For this review, use the dimensioned drawing (mm, ordinates from the lowest corner) and the shaded views. Round coordinates to 2 decimals unless told otherwise and drop trailing zeros. Loops run counter-clockwise (first coordinate to the right, second up) from the corner with the lowest first, then second, coordinate; pieces in that order, holes last. Notation, with made-up numbers: M 19,62 L 78,62 A16 cw 78,90 Z; hole C 2,-1.5 d10. An arc over 180 degrees is marked long. Answer as a JSON object with one key per item and string values. Group by question number.
Item 1: Consider section C-C (z = 2.7). Give the boundary of the cut face in (x, y).
Item 2: The part is to be moulded in two halves that separate along Y. For the marked faces 1 and 2, say which applies: +Y half, -Y half, draft (parallel to the pull), parting line (faces both ways), or undercut.
Item 3: Insertion check: P1, Ø1, axis at y = 35.5, z = 3.5, coming from the +X side; P2, Ø1, axis at y = 20, z = 1.5, coming from the -X side. Each pin has a flat end and moves straight along its axis. Give the tip position at first contact, or say it passes through.
Item 4: To check wall thickness, follow line 1 (Y direction, x = 7, z = 4.5); line 2 (X direction, y = 60, z = 3); line 3 (X direction, y = 47.5, z = 0.7). State the ranges of each line that lie inside material, in increasing order.
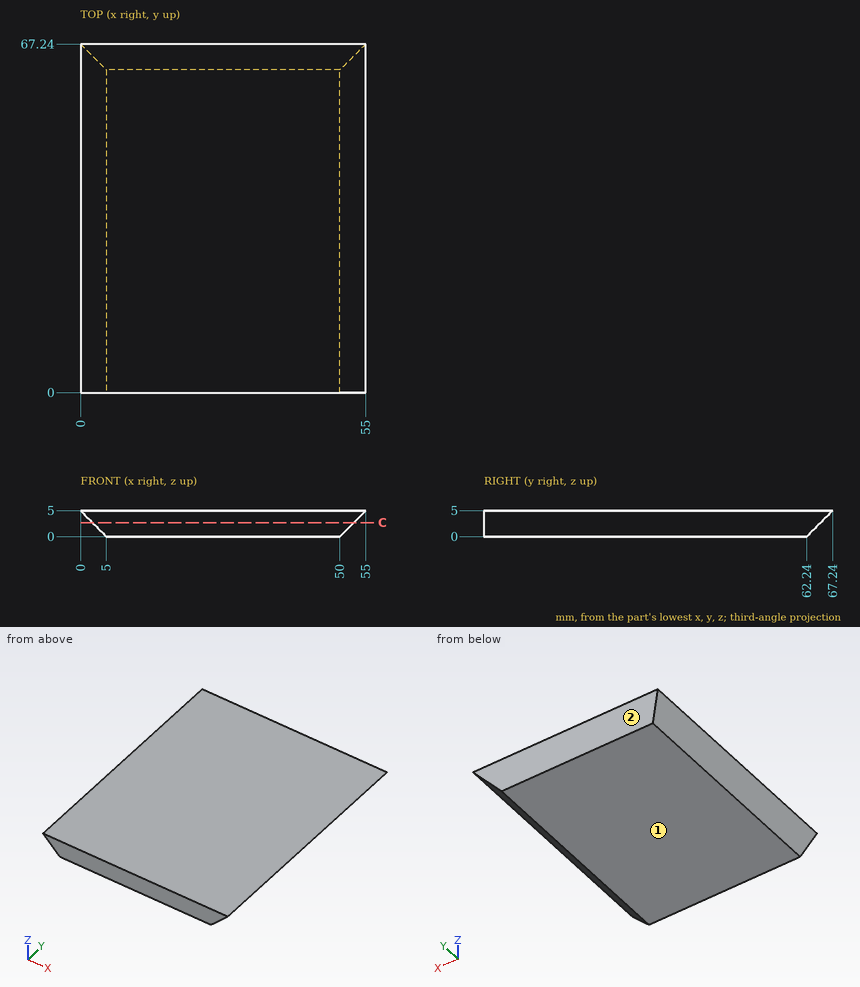
Geometry results:
{
 "1": {"outline": "M 2.3,0 L 52.7,0 L 52.7,64.94 L 2.3,64.94 Z"},
 "2": {"face 1": "draft", "face 2": "+Y half"},
 "3": {"P1": "stops at x = 54", "P2": "stops at x = 3"},
 "4": {"line 1": "y = 0 to 66.74", "line 2": "x = 2 to 53", "line 3": "x = 4.3 to 50.7"}
}
